from build123d import *

# Parameters (mm, degrees)
SKETCH_R           = 8
PAD_DEPTH          = 13
SKETCH001_R        = 3.05
PAD001_DEPTH       = 6
FILLET_R           = 2
SKETCH002_R        = 2.5
POCKET_DEPTH       = 52.192953
POCKET_DEPTH_BACK  = 65.192953
POLARPATTERN_COUNT = 8


with BuildPart() as part:
    # Sketch → Pad (new body)
    with BuildSketch(Plane.XY):
        Circle(SKETCH_R)
        with BuildLine():
            ThreePointArc((1.456056, 2.68), (-3.05, 0), (1.456056, -2.68))
            Line((1.456056, 2.68), (1.456056, -2.68))
        make_face(mode=Mode.SUBTRACT)
    extrude(amount=PAD_DEPTH)

    # Sketch001 (on Face5 of Pad) → Pad001 (join)
    with BuildSketch(Plane.XY.offset(13)):
        Circle(SKETCH001_R)
    extrude(amount=-PAD001_DEPTH)

    # Fillet
    fillet_edges = [part.edges().sort_by_distance(p)[0] for p in [
        (-8, 0, 13),
    ]]
    fillet(fillet_edges, radius=FILLET_R)

    # Sketch002 → Pocket (cut, two sides)
    with BuildSketch(Plane.XY) as pocket_sk:
        with Locations((0, 9.5)):
            Circle(SKETCH002_R)
    pocket = extrude(amount=-POCKET_DEPTH, mode=Mode.SUBTRACT) + extrude(pocket_sk.sketch, amount=POCKET_DEPTH_BACK, mode=Mode.SUBTRACT)

    # PolarPattern: Pocket ×8 about axis
    polarpattern_axis = Axis((0, 0, 0), (0, 0, 1))
    for i in range(1, POLARPATTERN_COUNT):
        add(pocket.rotate(polarpattern_axis, i * 360 / POLARPATTERN_COUNT), mode=Mode.SUBTRACT)


solid = part.part
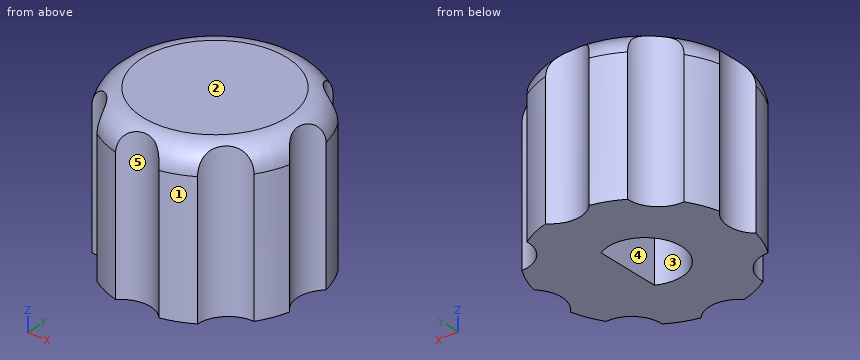
Part model, mm, in its own coordinate system. Face numbers are marked on the shaded views. A direction names the side the tool comes from. Give positions to 0.01 mm unless a question says otherwise; leave off trailing zeros. Loops run counter-clockwise (first coordinate to the right, second up) from the corner with the lowest first, then second, coordinate; pieces in that order, holes last. Notation, with made-up numbers: M 20,14 L 71,14 A27 cw 71,49 Z; hole C 33.25,78.25 d5. An arc over 180 degrees is marked long. Put each result on its own line as item: value. Start each with the question number.
1) Saw through at D-D (z = 10.5). List the corners of the cut face in (x, y), then the cut area to 3 significant figures.
2) Saw through at A-A (y = 0). List the corners of the cut face in (x, z).
3) Saw through at C-C (z = 4.5). List the corners of the cut face in (x, y).
4) Saw through at B-B (x = 0). List the corners of the cut face in (y, z).
5) Probe probe 1 along X at (y, z) = (0, 3); probe 2 along Y at (x, z) = (0, 4.25); probe 3 along Y at (x, z) = (-0.5, 5.75). List the from-to ranges inside material, lowest first.
6) Pull direction X, two halves, no side cores. Call the marked faces 1, 2 and 3: +X half, -X half, draft (parallel to the pull), parting line (faces both ways), or undercut.
7) 3-axis set-ups, long thin cutter, end or side, ignore diameter. For the marked faces 4 and 5: which of +Z, -Z, +X, -X, +Y, -Y reach the whole face in a straight line?
8) Flat gauge pins, fed straight in: pin 1 (1.5 mm diameter, centred on x = 4.5, z = 3.5, fed in from -Y); pin 2 (1.6 mm diameter, centred on y = -0.5, z = 3, fed in from -X); pin 3 (1.4 mm diameter, centred on x = -1, y = 0, fed in from -Z). Where does each tip first touch, or does it go through?
Numbers:
1. outline: M -7.79,-1.82 A8 ccw -6.8,-4.22 A2.5 cw -4.22,-6.8 A8 ccw -1.82,-7.79 A2.5 cw 1.82,-7.79 A8 ccw 4.22,-6.8 A2.5 cw 6.8,-4.22 A8 ccw 7.79,-1.82 A2.5 cw 7.79,1.82 A8 ccw 6.8,4.22 A2.5 cw 4.22,6.8 A8 ccw 1.82,7.79 A2.5 cw -1.82,7.79 A8 ccw -4.22,6.8 A2.5 cw -6.8,4.22 A8 ccw -7.79,1.82 A2.5 cw Z
1. area: 181 mm^2
2. outline: M -7,0 L -3.05,0 L -3.05,7 L 1.46,7 L 1.46,0 L 7,0 L 7,12.73 A2 ccw 6,13 L -6,13 A2 ccw -7,12.73 Z
3. outline: M -7.79,-1.82 A8 ccw -6.8,-4.22 A2.5 cw -4.22,-6.8 A8 ccw -1.82,-7.79 A2.5 cw 1.82,-7.79 A8 ccw 4.22,-6.8 A2.5 cw 6.8,-4.22 A8 ccw 7.79,-1.82 A2.5 cw 7.79,1.82 A8 ccw 6.8,4.22 A2.5 cw 4.22,6.8 A8 ccw 1.82,7.79 A2.5 cw -1.82,7.79 A8 ccw -4.22,6.8 A2.5 cw -6.8,4.22 A8 ccw -7.79,1.82 A2.5 cw Z; hole M 1.46,-2.68 L 1.46,2.68 A3.05 ccw long Z
4. outline: M -7,0 L -3.05,0 L -3.05,7 L 3.05,7 L 3.05,0 L 7,0 L 7,12.73 A2 ccw 6,13 L -6,13 A2 ccw -7,12.73 Z
5. probe 1: -7 to -3.05, 1.46 to 7
5. probe 2: -7 to -3.05, 3.05 to 7
5. probe 3: -7.05 to -3.01, 3.01 to 7.05
6. face 1: +X half
6. face 2: draft
6. face 3: undercut
7. face 4: -Z
7. face 5: +Z, -Z, -Y
8. pin 1: y = -7.07
8. pin 2: x = -7.36
8. pin 3: z = 7
